Here's how the part is built. I have some questions about the finished solid (model axes, mm). Face numbers are marked on the shaded views. Round coordinates to 2 decimals unless told otherwise and drop trailing zeros. Loops run counter-clockwise (first coordinate to the right, second up) from the corner with the lowest first, then second, coordinate; pieces in that order, holes last. Notation, with made-up numbers: M -36.5,29.5 L -17.5,29.5 A18 cw -17.5,50.5 Z; hole C 30,48 d6. An arc over 180 degrees is marked long. Write item = value, one per line. Start each with the question number.
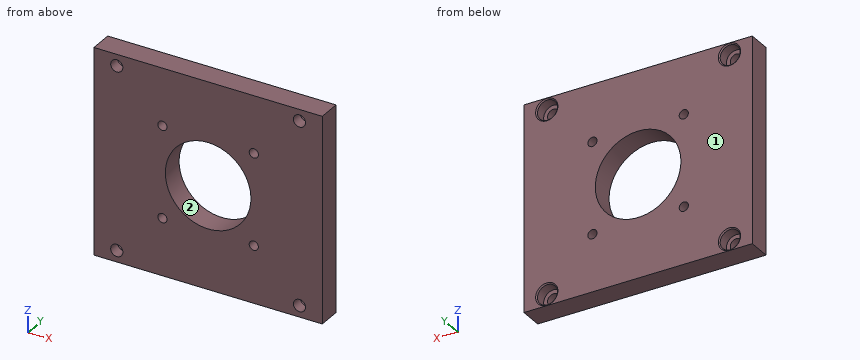
from build123d import *

# Parameters (mm, degrees)
SKETCH1_W                                     = 127
SKETCH1_H                                     = 114.3
BOSS_EXTRUDE1_DEPTH                           = 12.7
SKETCH2_R                                     = 23.8125
CUT_EXTRUDE1_DEPTH                            = 87.36933773
CBORE_FOR_1_4_SOCKET_HEAD_CAP_SCREW1_AT_COUNT = 2
CBORE_FOR_1_4_SOCKET_HEAD_CAP_SCREW1_AT_PITCH = 101.6
CBORE_FOR_1_4_SOCKET_HEAD_CAP_SCREW1_2_COUNT  = 2
CBORE_FOR_1_4_SOCKET_HEAD_CAP_SCREW1_2_PITCH  = 143.684097937
CBORE_FOR_1_4_SOCKET_HEAD_CAP_SCREW1_3_COUNT  = 2
CBORE_FOR_1_4_SOCKET_HEAD_CAP_SCREW1_3_PITCH  = 101.6
F_1_4_20_TAPPED_HOLE1_D                       = 5.1054
F_1_4_20_TAPPED_HOLE1_DEPTH                   = 16.51
F_1_4_20_TAPPED_HOLE1_TIP                     = 1.533816902


with BuildPart() as part:
    # Sketch1 → Boss-Extrude1 (new body)
    with BuildSketch(Plane(origin=(0, 0, 0), x_dir=(1, 0, 0), z_dir=(0, 1, 0))):
        Rectangle(SKETCH1_W, SKETCH1_H)
    extrude(amount=BOSS_EXTRUDE1_DEPTH)

    # Sketch2 → Cut-Extrude1 (cut, through all)
    with BuildSketch(Plane(origin=(0, 12.7, 0), x_dir=(1, 0, 0), z_dir=(0, 1, 0))):
        with Locations(Location((0, 0, 0), (0, 0, 270))):
            Circle(SKETCH2_R)
    extrude(amount=-CUT_EXTRUDE1_DEPTH, mode=Mode.SUBTRACT)

    # Sketch5 → CBORE for 1/4 Socket Head Cap Screw1 (revolve, cut)
    with BuildSketch(Plane(origin=(-50.8, 12.7, -50.8), x_dir=(0, 0, 1), z_dir=(1, 0, 0))):
        Polygon((0, 0), (0, 12.7), (3.3782, 12.7), (3.3782, 6.35), (5.55625, 6.35), (5.55625, 0.635), (6.19125, 0), align=None)
    cbore_for_1_4_socket_head_cap_screw1 = revolve(axis=Axis((-50.8, 19.05, -50.8), (0, -1, 0)), mode=Mode.SUBTRACT)

    # CBORE for 1/4 Socket Head Cap Screw1 at: CBORE for 1/4 Socket Head Cap Screw1 ×2
    with Locations(*[(i * CBORE_FOR_1_4_SOCKET_HEAD_CAP_SCREW1_AT_PITCH, 0, 0) for i in range(1, CBORE_FOR_1_4_SOCKET_HEAD_CAP_SCREW1_AT_COUNT)]):
        add(cbore_for_1_4_socket_head_cap_screw1, mode=Mode.SUBTRACT)

    # CBORE for 1_4 Socket Head Cap Screw1 2: CBORE for 1/4 Socket Head Cap Screw1 ×2
    with Locations(*[Vector(0.7071067811865476, 0, 0.7071067811865475) * (i * CBORE_FOR_1_4_SOCKET_HEAD_CAP_SCREW1_2_PITCH) for i in range(1, CBORE_FOR_1_4_SOCKET_HEAD_CAP_SCREW1_2_COUNT)]):
        add(cbore_for_1_4_socket_head_cap_screw1, mode=Mode.SUBTRACT)

    # CBORE for 1_4 Socket Head Cap Screw1 3: CBORE for 1/4 Socket Head Cap Screw1 ×2
    with Locations(*[(0, 0, i * CBORE_FOR_1_4_SOCKET_HEAD_CAP_SCREW1_3_PITCH) for i in range(1, CBORE_FOR_1_4_SOCKET_HEAD_CAP_SCREW1_3_COUNT)]):
        add(cbore_for_1_4_socket_head_cap_screw1, mode=Mode.SUBTRACT)

    # 1/4-20 Tapped Hole1
    with Locations(Plane(origin=(-25.4, 12.7, -25.4), x_dir=(0, 0, 1), z_dir=(0, 1, 0))):
        with Locations((0, 0), (0, 50.8), (50.8, 50.8), (50.8, 0)):
            Hole(F_1_4_20_TAPPED_HOLE1_D / 2, depth=F_1_4_20_TAPPED_HOLE1_DEPTH)
            with Locations((0, 0, -(F_1_4_20_TAPPED_HOLE1_DEPTH + F_1_4_20_TAPPED_HOLE1_TIP / 2))):  # 118° drill point
                Cone(0, F_1_4_20_TAPPED_HOLE1_D / 2, F_1_4_20_TAPPED_HOLE1_TIP, mode=Mode.SUBTRACT)


solid = part.part
Item 1: I want a section at B-B, the plane z = 25.4. List the corners of the cut face in (x, y) for me.
Item 2: I want a section at D-D, the plane z = -5. List the corners of the cut face in (x, y) for me, then the cut area to 3 significant figures.
Item 3: Please list where these lines run through material, in increasing order: line 1 (Z direction, x = -50.8, y = 9.35); line 2 (X direction, y = 8, z = 25.4); line 3 (X direction, y = 3, z = 50.8). Write a range as [from, to].
Item 4: I want a section at C-C, the plane y = 2. State how many separate pieces and enclosed holes the cut face has, then the cut area to 3 significant figures.
Item 5: We'd pull the mould along Z, two halves only. Please class the marked faces 1 and 2: released by +Z, released by -Z, zero draft, split by the parting line, or undercut.
Item 6: I want a section at A-A, the plane x = 25.4. List the corners of the cut face in (y, z) for me.
Item 7: Will these pins go through, and if not, where does the flat tip stop? pin 1 Ø9 at (x, z) = (-50.5, -50.5) entering from +Y; pin 2 Ø6 at (x, z) = (50.8, 50.8) entering from +Y.
Worked out:
q1.outline = M -63.5,0 L -27.95,0 L -27.95,12.7 L -63.5,12.7 Z; M -22.85,0 L 22.85,0 L 22.85,12.7 L -22.85,12.7 Z; M 27.95,0 L 63.5,0 L 63.5,12.7 L 27.95,12.7 Z
q2.outline = M -63.5,0 L -23.28,0 L -23.28,12.7 L -63.5,12.7 Z; M 23.28,0 L 63.5,0 L 63.5,12.7 L 23.28,12.7 Z
q2.area = 1,020 mm2
q3.line_1 = [-57.15, -56.36], [-45.24, 45.24], [56.36, 57.15]
q3.line_2 = [-63.5, -27.95], [-22.85, 22.85], [27.95, 63.5]
q3.line_3 = [-63.5, -54.18], [-47.42, 47.42], [54.18, 63.5]
q4.separate_pieces = 1
q4.enclosed_holes = 9
q4.area = 12,500 mm2
q5.face_1 = zero draft
q5.face_2 = undercut
q6.outline = M 0,-57.15 L 12.7,-57.15 L 12.7,-27.95 L 0,-27.95 Z; M 0,-22.85 L 12.7,-22.85 L 12.7,22.85 L 0,22.85 Z; M 0,27.95 L 12.7,27.95 L 12.7,57.15 L 0,57.15 Z
q7.pin_1 = 6.35
q7.pin_2 = through
